Verification items for the finished model (mm, model axes). Face numbers are marked on the shaded views. A direction names the side the tool comes from. Coordinates: 2 decimals unless noted, no trailing zeros. Order: outer loops, then holes, each group sorted by start corner. A loop starts at its lowest first (then second) coordinate and runs counter-clockwise, first axis right, second up.
Q1. Thickness scan on line 1 (X direction, y = 3, z = 0); line 2 (Y direction, x = -4, z = -4.25); line 3 (Z direction, x = 0, y = -0.1). Record the ranges inside material, lowest first.
Q2. Cross-section at B-B, the plane z = 0. Record the boundary of the cut face in (x, y), and give its area (3 significant figures).
Q3. Set-up check for the marked faces 1, 2 and 3: record each of +Z, -Z, +X, -X, +Y, -Y from which the full face is reachable in a straight line by a thin tool's end or side.
Q4. Depth check by flat-ended pin: P1, Ø2, axis at x = -0.5, y = 2, coming from the -Z side; P2, Ø5, axis at x = 0, z = 0, coming from the +Y side; P3, Ø1.5, axis at y = 3.5, z = -4.5, coming from the -X side. Enter the tip coordinate at first touch or a pass-through.
Q5. Draft check along Y on the marked faces 4, 5, 6 and 7. Enter one of: pulls with the +Y half, pulls with the -Y half, needs draft (parallel to the pull), parting line crosses it, or undercut.
Q6. Cross-section at C-C, the plane y = 2. Record the boundary of the cut face in (x, z).
Q7. Cross-section at D-D, the plane x = -2.75. Record the boundary of the cut face in (y, z).
Q8. Cross-section at A-A, the plane x = 0. Record the boundary of the cut face in (y, z), and give its area (3 significant figures).
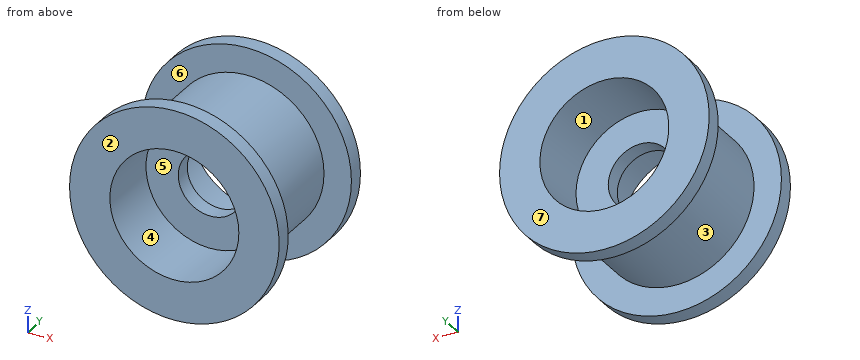
from build123d import *

# Parameters (mm, degrees)
SKETCH2_R           = 4.8
BOSS_EXTRUDE1_DEPTH = 3.5
SKETCH3_R           = 6.5
BOSS_EXTRUDE2_DEPTH = 1
SKETCH4_R           = 4
CUT_EXTRUDE1_DEPTH  = 4
SKETCH5_R           = 2
CUT_EXTRUDE2_DEPTH  = 6


with BuildPart() as part:
    # Sketch2 → Boss-Extrude1 (new body, symmetric)
    with BuildSketch(Plane(origin=(0, 0, 0), x_dir=(1, 0, 0), z_dir=(0, 1, 0))):
        Circle(SKETCH2_R)
    extrude(amount=BOSS_EXTRUDE1_DEPTH, both=True)

    # Sketch3 → Boss-Extrude2 (add)
    with BuildSketch(Plane(origin=(0, 3.5, 0), x_dir=(1, 0, 0), z_dir=(0, 1, 0))):
        Circle(SKETCH3_R)
    boss_extrude2 = extrude(amount=BOSS_EXTRUDE2_DEPTH)

    # Sketch4 → Cut-Extrude1 (cut)
    with BuildSketch(Plane(origin=(0, 4.5, 0), x_dir=(1, 0, 0), z_dir=(0, 1, 0))):
        Circle(SKETCH4_R)
    cut_extrude1 = extrude(amount=-CUT_EXTRUDE1_DEPTH, mode=Mode.SUBTRACT)

    # Mirror1: Boss-Extrude2, Cut-Extrude1 across plane
    add(boss_extrude2.mirror(Plane.ZX))
    add(cut_extrude1.mirror(Plane.ZX), mode=Mode.SUBTRACT)

    # Sketch5 → Cut-Extrude2 (cut, through all)
    with BuildSketch(Plane(origin=(0, 0.5, 0), x_dir=(1, 0, 0), z_dir=(0, 1, 0))):
        Circle(SKETCH5_R)
    extrude(amount=-CUT_EXTRUDE2_DEPTH, mode=Mode.SUBTRACT)


solid = part.part
Check values:
1. line 1: x = -4.8 to -4, 4 to 4.8
1. line 2: y = -4.5 to -3.5, 3.5 to 4.5
1. line 3: z = -4.8 to -2, 2 to 4.8
2. outline: (-6.5, -4.5) - (-4, -4.5) - (-4, -0.5) - (-2, -0.5) - (-2, 0.5) - (-4, 0.5) - (-4, 4.5) - (-6.5, 4.5) - (-6.5, 3.5) - (-4.8, 3.5) - (-4.8, -3.5) - (-6.5, -3.5) - close; (2, -0.5) - (4, -0.5) - (4, -4.5) - (6.5, -4.5) - (6.5, -3.5) - (4.8, -3.5) - (4.8, 3.5) - (6.5, 3.5) - (6.5, 4.5) - (4, 4.5) - (4, 0.5) - (2, 0.5) - close
2. area: 25.2 mm2
3. face 1: +Y
3. face 2: +Z, -Z, +X, -X, -Y
3. face 3: none
4. P1: stops at z = -4.8
4. P2: stops at y = 0.5
4. P3: stops at x = -5.31
5. face 4: needs draft
5. face 5: pulls with the -Y half
5. face 6: undercut
5. face 7: pulls with the +Y half
6. outline: circle Ø9.6 at (0, 0); hole circle Ø8 at (0, 0)
7. outline: (-4.5, -5.89) - (-3.5, -5.89) - (-3.5, -3.93) - (3.5, -3.93) - (3.5, -5.89) - (4.5, -5.89) - (4.5, -2.9) - (0.5, -2.9) - (0.5, 2.9) - (4.5, 2.9) - (4.5, 5.89) - (3.5, 5.89) - (3.5, 3.93) - (-3.5, 3.93) - (-3.5, 5.89) - (-4.5, 5.89) - (-4.5, 2.9) - (-0.5, 2.9) - (-0.5, -2.9) - (-4.5, -2.9) - close
8. outline: (-4.5, -6.5) - (-3.5, -6.5) - (-3.5, -4.8) - (3.5, -4.8) - (3.5, -6.5) - (4.5, -6.5) - (4.5, -4) - (0.5, -4) - (0.5, -2) - (-0.5, -2) - (-0.5, -4) - (-4.5, -4) - close; (-4.5, 4) - (-0.5, 4) - (-0.5, 2) - (0.5, 2) - (0.5, 4) - (4.5, 4) - (4.5, 6.5) - (3.5, 6.5) - (3.5, 4.8) - (-3.5, 4.8) - (-3.5, 6.5) - (-4.5, 6.5) - close
8. area: 25.2 mm2
